Answer from the drawing. Dimensions are ordinates in mm from the lowest x, y and z of the part. A direction names the side the tool comes from. Give positions to 0.01 mm unless a question says otherwise; leave off trailing zeros. Order: outer loops, then holes, each group sorted by start corner. A loop starts at its lowest first (then second) coordinate and runs counter-clockwise, first axis right, second up. Notation, with made-up numbers: (26, -1.75) - (68, -1.75) arc R18 cw to (68, 15.25) - close; hole circle Ø10 at (73.25, 28.5). An arc over 180 degrees is marked (long way). Use a Markdown table: item, result. Add a question column.
1) Find section D-D, the plane x = 5.5. Determine the outline of the cut face in (y, z).
2) Find section B-B, the plane z = 21.5. Determine the outline of the cut face in (x, y) (1 decimal), plus the area to 3 significant figures.
3) Find section C-C, the plane y = 20.5. Determine the outline of the cut face in (x, z) (1 decimal).
4) Straight lines are drawn through the part: line 1 (Y direction, x = 8.25, z = 9); line 2 (Z direction, x = 1.75, y = 20) (1 decimal); line 3 (Z direction, x = 6, y = 29). For each, find the intervals that lie inside material, in ascending order.
5) The mould has two halves that part along Z. Classify the marked faces 4, 5 and 6: released by +Z, released by -Z, zero draft, split by the parting line, or undercut.
6) Find section A-A, the plane x = 9.5. State how many separate pieces and enclosed holes the cut face has.
7) Flat-ended cylindrical pins translate along their axes: pin 1 (7 mm diameter, centred on x = 8.5, y = 19.5, fed in from +Z); pin 2 (3 mm diameter, centred on x = 2, y = 23.5, fed in from -Z); pin 3 (1 mm diameter, centred on x = 3.5, z = 7.5, fed in from +Y). Find the tip coordinate at first contact, or state that the pin passes through.
8) For the marked faces 1, 2 and 3, determine the directions among +Z, -Z, +X, -X, +Y, -Y from which every point of the face is accessible in a straight line to the end or side of a thin tool.
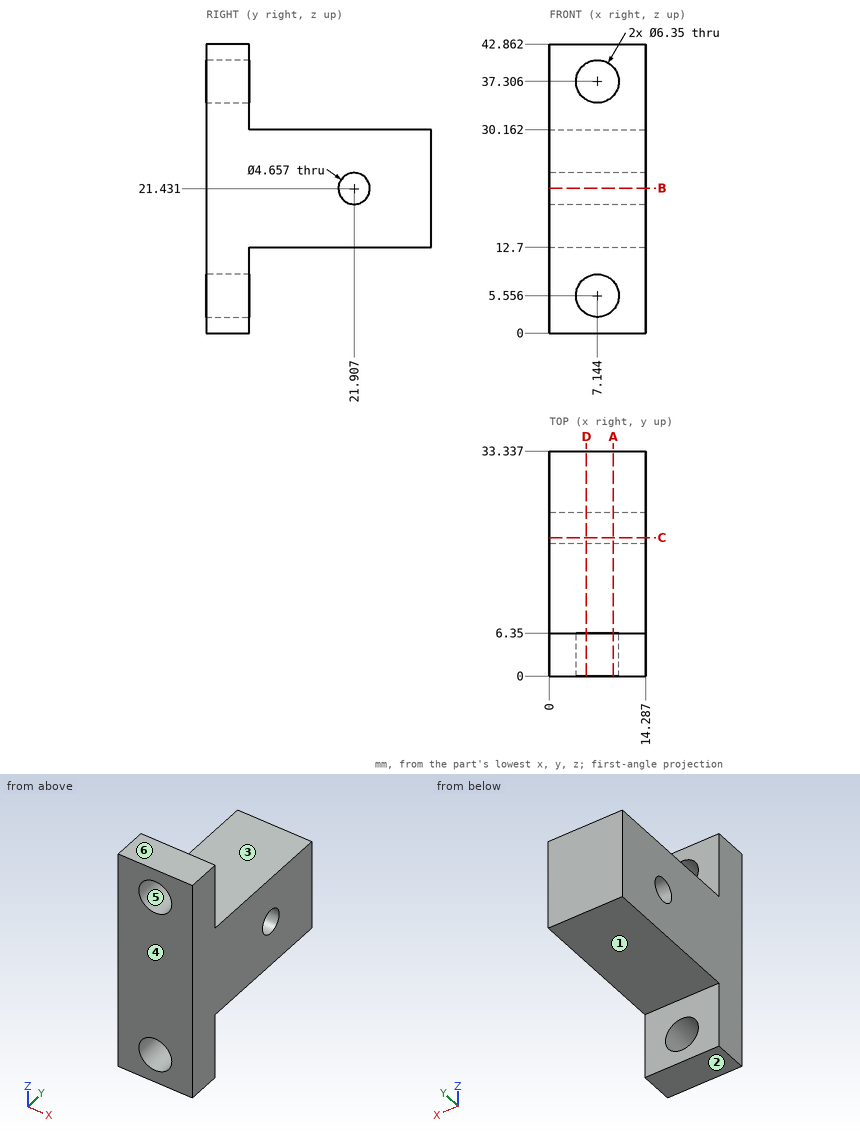
The answers:
| question | item | result |
|---|---|---|
| 1 | outline | (0, 0) - (6.35, 0) - (6.35, 2.84) - (0, 2.84) - close; (0, 8.27) - (6.35, 8.27) - (6.35, 12.7) - (33.34, 12.7) - (33.34, 30.16) - (6.35, 30.16) - (6.35, 34.59) - (0, 34.59) - close; (0, 40.02) - (6.35, 40.02) - (6.35, 42.86) - (0, 42.86) - close; hole circle Ø4.66 at (21.91, 21.43) |
| 2 | outline | (0, 0) - (14.3, 0) - (14.3, 19.6) - (0, 19.6) - close; (0, 24.2) - (14.3, 24.2) - (14.3, 33.3) - (0, 33.3) - close |
| 2 | area | 410 mm2 |
| 3 | outline | (0, 12.7) - (14.3, 12.7) - (14.3, 19.6) - (0, 19.6) - close; (0, 23.3) - (14.3, 23.3) - (14.3, 30.2) - (0, 30.2) - close |
| 4 | line 1 | 0 to 6.35 |
| 4 | line 2 | 12.7 to 20.1, 22.8 to 30.2 |
| 4 | line 3 | 12.7 to 30.16 |
| 5 | face 4 | zero draft |
| 5 | face 5 | undercut |
| 5 | face 6 | released by +Z |
| 6 | separate pieces | 3 |
| 6 | enclosed holes | 1 |
| 7 | pin 1 | z = 30.16 |
| 7 | pin 2 | z = 12.7 |
| 7 | pin 3 | y = 6.35 |
| 8 | face 1 | -Z, +X, -X, +Y |
| 8 | face 2 | -Z, +X, -X, +Y, -Y |
| 8 | face 3 | +Z, +X, -X, +Y |
